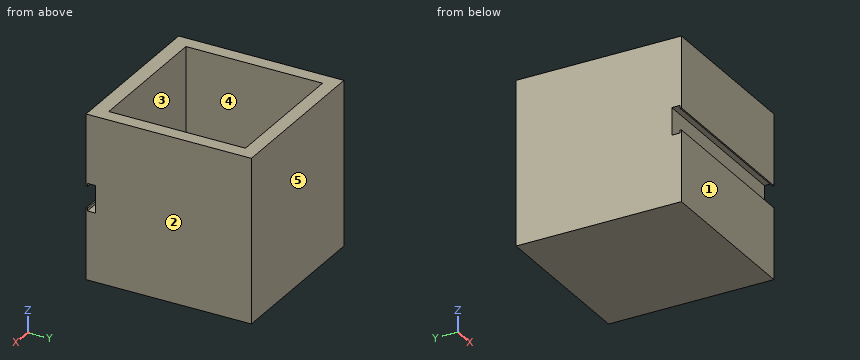
Autodesk Fusion 360 part; units mm, degrees
sketch "Sketch1" plane through (0, 0, 0) normal (0, 0, 1) x (1, 0, 0)
  line L0 (50.6391, 82.0886) -> (110.6391, 82.0886)
  line L1 (110.6391, 82.0886) -> (110.6391, 22.0886)
  line L2 (110.6391, 22.0886) -> (50.6391, 22.0886)
  line L3 (50.6391, 22.0886) -> (50.6391, 82.0886)
  line L4 (55.6391, 77.0886) -> (105.6391, 77.0886)
  line L5 (105.6391, 77.0886) -> (105.6391, 27.0886)
  line L6 (105.6391, 27.0886) -> (55.6391, 27.0886)
  line L7 (55.6391, 27.0886) -> (55.6391, 77.0886)
  dimension "d1" = 60
  dimension "d2" = 60
  dimension "d5" = 50
  dimension "d6" = 50
extrude "Extrude1" add sketch "Sketch1" along normal blind 10 contours L4 L5 L6 L7
extrude "Extrude2" add sketch "Sketch1" along normal blind 60
sketch "Sketch2" plane through (0, 22.0886, 0) normal (0, -1, 0) x (1, 0, 0)
  line L0 (50.6391, 0) -> (110.6391, 0)
  line L1 (110.6391, 0) -> (110.6391, 60)
  line L2 (110.6391, 60) -> (50.6391, 60)
  line L3 (50.6391, 60) -> (50.6391, 0)
  line L4 (80.6391, 35) -> (75.6391, 35)
  line L5 (75.6391, 35) -> (85.6391, 35)
  line L6 (85.6391, 35) -> (85.6391, 25)
  line L7 (85.6391, 25) -> (75.6391, 25)
  line L8 (75.6391, 25) -> (75.6391, 35)
  dimension "d13" = 10
  dimension "d14" = 10
extrude "Extrude3" cut sketch "Sketch2" against normal blind 3.3 contours L4 L5 L6 L7 L8
extrude "Extrude4" add 1 faces at (78.9724, 25.3886, 31.6667) along direction (0, -1, 0) blind 3.3
sketch "Sketch3" plane through (0, 22.0886, 0) normal (0, -1, 0) x (1, 0, 0)
  line L0 (50.6391, 0) -> (110.6391, 0)
  line L1 (110.6391, 0) -> (110.6391, 60)
  line L2 (110.6391, 60) -> (50.6391, 60)
  line L3 (50.6391, 60) -> (50.6391, 0)
extrude "Extrude5" add 1 faces at (70.6391, 22.0886, 40) along direction (0, -1, 0) blind 0.5
sketch "Sketch4" plane through (110.6391, 0, 0) normal (1, 0, 0) x (0, 1, 0)
  line L0 (21.5886, 0) -> (82.0886, 0)
  line L1 (82.0886, 0) -> (82.0886, 60)
  line L2 (82.0886, 60) -> (21.5886, 60)
  line L3 (21.5886, 60) -> (21.5886, 0)
  line L4 (22.0886, 30) -> (22.0886, 35)
  line L5 (22.0886, 35) -> (25.0886, 35)
  line L6 (25.0886, 35) -> (25.0886, 25)
  line L7 (25.0886, 25) -> (22.0886, 25)
  line L8 (22.0886, 25) -> (22.0886, 35)
  line L9 (22.0886, 35) -> (22.0886, 34)
  line L10 (22.0886, 34) -> (21.5886, 34)
  line L11 (21.5886, 34) -> (21.5886, 26)
  line L12 (21.5886, 26) -> (22.0886, 26)
  line L13 (22.0886, 26) -> (22.0886, 34)
  dimension "d22" = 5
  dimension "d23" = 3
  dimension "d24" = 10
  dimension "d25" = 1
  dimension "d26" = 8
extrude "Extrude6" cut sketch "Sketch4" against normal blind 60 contours L3 L4 L8 L10 L11 L12 L13 | L4 L5 L6 L7 L8 L9 L13
Read the model definition and answer for the solid it produces. Units are mm, in the model's axes. Face numbers are marked on the shaded views. A direction names the side the tool comes from. Round coordinates to 2 decimals unless told otherwise and drop trailing zeros. Loops run counter-clockwise (first coordinate to the right, second up) from the corner with the lowest first, then second, coordinate; pieces in that order, holes last.
Q1. Section A-A on z = 41 is taken. Write down the section's boundary in (x, y), and give its area (3 significant figures).
Q2. Section C-C on x = 59.5 is taken. Write down the section's boundary in (y, z).
Q3. Section B-B on y = 51.5 is taken. Write down the section's boundary in (x, z).
Q4. Determine the mould class of the marked faces 1, 2 and 3 for opening direction X: released by +X, released by -X, zero draft, split by the parting line, or undercut.
Q5. Consider probe 1 along X at (y, z) = (76.5, 54.5); probe 2 along Y at (x, z) = (70.5, 49); probe 3 along Y at (x, z) = (84.5, 33.5). Determine where each line is inside the solid, lowest interval first.
Q6. This flat-tipped pin is pushed along its axis until it touches: pin 1 (15 mm diameter, centred on x = 89, y = 44.5, fed in from +Z). Where does it stop, or does it pass through?
Q7. Which of the six approach directions +Z, -Z, +X, -X, +Y, -Y give full straight-line access (tool end or side, diameter ignored) to the marked faces 4 and 5?
Output:
1. outline: (50.64, 21.59) - (110.64, 21.59) - (110.64, 82.09) - (50.64, 82.09) - close; hole (55.64, 27.09) - (105.64, 27.09) - (105.64, 77.09) - (55.64, 77.09) - close
1. area: 1,130 mm2
2. outline: (21.59, 0) - (82.09, 0) - (82.09, 60) - (77.09, 60) - (77.09, 10) - (27.09, 10) - (27.09, 60) - (21.59, 60) - (21.59, 34) - (22.09, 34) - (22.09, 35) - (25.09, 35) - (25.09, 25) - (22.09, 25) - (22.09, 26) - (21.59, 26) - close
3. outline: (50.64, 0) - (110.64, 0) - (110.64, 60) - (105.64, 60) - (105.64, 10) - (55.64, 10) - (55.64, 60) - (50.64, 60) - close
4. face 1: zero draft
4. face 2: released by +X
4. face 3: undercut
5. probe 1: x = 50.64 to 55.64, 105.64 to 110.64
5. probe 2: y = 21.59 to 27.09, 77.09 to 82.09
5. probe 3: y = 25.09 to 27.09, 77.09 to 82.09
6. pin 1: stops at z = 10
7. face 4: +Z
7. face 5: +Z, -Z, +X, -X, +Y
